from build123d import *

# Parameters (mm, degrees)
SKETCH1_W           = 41.275
SKETCH1_H           = 44.45
BOSS_EXTRUDE1_DEPTH = 3.175
FILLET1_R           = 3.175
SKETCH2_R           = 3.175
SKETCH2_R_2         = 3.561696706
CUT_EXTRUDE1_DEPTH  = 61.741326541


with BuildPart() as part:
    # Sketch1 → Boss-Extrude1 (new body)
    with BuildSketch(Plane(origin=(0, 0, 0), x_dir=(1, 0, 0), z_dir=(0, 1, 0))):
        with Locations((20.6375, 22.225)):
            Rectangle(SKETCH1_W, SKETCH1_H)
    extrude(amount=BOSS_EXTRUDE1_DEPTH)

    # Fillet1
    fillet1_edges = [part.edges().sort_by_distance(p)[0] for p in [
        (0, 1.5875, -44.45),
        (41.275, 1.5875, -44.45),
        (41.275, 1.5875, 0),
        (0, 1.5875, 0),
    ]]
    fillet(fillet1_edges, radius=FILLET1_R)

    # Sketch2 → Cut-Extrude1 (cut, through all)
    with BuildSketch(Plane(origin=(0, 3.175, 0), x_dir=(1, 0, 0), z_dir=(0, 1, 0))):
        with Locations(Location((9.525, 36.5125, 0), (0, 0, 270))):
            Circle(SKETCH2_R)
        with Locations(Location((31.75, 36.5125, 0), (0, 0, 270))):
            Circle(SKETCH2_R_2)
        with Locations(Location((20.6375, 12.7, 0), (0, 0, 270))):
            Circle(SKETCH2_R)
    extrude(amount=-CUT_EXTRUDE1_DEPTH, mode=Mode.SUBTRACT)


solid = part.part
The model under review builds one solid part; all positions refer to its coordinate system, in mm. Give positions to 0.01 mm unless a question says otherwise; leave off trailing zeros. Loops run counter-clockwise (first coordinate to the right, second up) from the corner with the lowest first, then second, coordinate; pieces in that order, holes last. Notation, with made-up numbers: (22, -9) -> (64, -9) arc R13 cw to (64, 0) -> close; hole circle Ø2 at (26.5, -25.5). An arc over 180 degrees is marked (long way). Write each question's results on one line, items separated by ' | '.
1) Draft analysis for pull direction X (two halves, no side actions). For faces 1 (the face through (21.59, 1.61, -9.67)), 2 (the face through (20, 0, -23)), 3 (the face through (35.28, 1.61, -36.98)), 4 (the face through (40.37, 1.61, -43.495)), state which applies: pulls with the +X half, pulls with the -X half, needs draft (parallel to the pull), parting line crosses it, or undercut.
Conclusion:
face 1: undercut | face 2: needs draft | face 3: undercut | face 4: pulls with the +X half
2) Take a section at B-B, the plane z = -12.7. Give the boundary of the cut face in (x, y) (1 decimal).
Conclusion:
outline: (0, 0) -> (17.5, 0) -> (17.5, 3.2) -> (0, 3.2) -> close; (23.8, 0) -> (41.3, 0) -> (41.3, 3.2) -> (23.8, 3.2) -> close
3) Take a section at D-D, the plane z = -38.5. Give the boundary of the cut face in (x, y) (3 decimals), plus the area to 3 significant figures.
Conclusion:
outline: (0, 0) -> (7.049, 0) -> (7.049, 3.175) -> (0, 3.175) -> close; (12.001, 0) -> (28.794, 0) -> (28.794, 3.175) -> (12.001, 3.175) -> close; (34.706, 0) -> (41.275, 0) -> (41.275, 3.175) -> (34.706, 3.175) -> close | area: 96.6 mm^2
4) Take a section at A-A, the plane x = 31.75. Give the boundary of the cut face in (y, z) (3 decimals).
Conclusion:
outline: (0, -44.45) -> (3.175, -44.45) -> (3.175, -40.074) -> (0, -40.074) -> close; (0, -32.951) -> (3.175, -32.951) -> (3.175, 0) -> (0, 0) -> close
5) Take a section at C-C, the plane y = 0.8. Count the separate pieces of the cut face and the enclosed holes in it, plus the area to 3 significant figures.
Conclusion:
separate pieces: 1 | enclosed holes: 3 | area: 1,720 mm^2
6) Insertion check: pin 1 Ø8.5 at (x, z) = (20.64, -12.7) entering from +Y (3 decimals); pin 2 Ø5 at (x, z) = (9.52, -36.51) entering from +Y. Each pin has a flat end and moves straight along its axis. Give the tip position at first contact, or say it passes through.
Conclusion:
pin 1: stops at y = 3.175 | pin 2: passes through
7) For line 1 along X through (y, z) = (2.4, -12.7) (1 decimal); line 2 along Z through (x, y) = (20, 0.25); line 3 along X through (y, z) = (2.9, -11.5) (3 decimals), list the stretches that pass through material, from the lowest coordinate up. Write a range as from..to.
Conclusion:
line 1: x = 0..17.5, 23.8..41.3 | line 2: z = -44.45..-15.81, -9.59..0 | line 3: x = 0..17.698, 23.577..41.275
